```python
from build123d import *

# Parameters (mm, degrees)
SKETCH1_R               = 2.85
SKETCH1_R_2             = 1.6
BOSS_EXTRUDE1_DEPTH     = 6.5
SKETCH1_3_R             = 2.85
SKETCH1_3_R_2           = 1.6
BOSS_EXTRUDE2_DEPTH     = 3
CUT_EXTRUDE1_START      = -3
SKETCH1_4_R             = 2.85
CUT_EXTRUDE1_DEPTH      = 3.5
CUT_EXTRUDE1_DEPTH_BACK = 4


with BuildPart() as part:
    # Sketch1 → Boss-Extrude1 (new body)
    with BuildSketch(Plane(origin=(0, 0, 0), x_dir=(0, 1, 0), z_dir=(0, 0, 1))):
        Polygon((-7.9, 10.1), (-9.9, 10.1), (-9.9, 0), (-9.1, 0), (-9.1, -2), (-20.1, -2), (-20.1, 11.6), (-7.9, 11.6), align=None)
        with Locations((-14.9, 6.1)):
            Circle(SKETCH1_R, mode=Mode.SUBTRACT)
        Polygon((13.4, 11.6), (20.1, 11.6), (20.1, -2), (9.1, -2), (9.1, 0), (9.9, 0), (9.9, 9.3), (6.4, 9.3), (6.4, 10.8), (13.4, 10.8), align=None)
        with Locations((14.9, 6.1)):
            Circle(SKETCH1_R, mode=Mode.SUBTRACT)
        with Locations((-14.9, 6.1)):
            Circle(SKETCH1_R)
        with Locations((-14.9, 6.1)):
            Circle(SKETCH1_R_2, mode=Mode.SUBTRACT)
        with Locations((14.9, 6.1)):
            Circle(SKETCH1_R)
        with Locations((14.9, 6.1)):
            Circle(SKETCH1_R_2, mode=Mode.SUBTRACT)
    extrude(amount=BOSS_EXTRUDE1_DEPTH)

    # Sketch1<3> → Boss-Extrude2 (add)
    with BuildSketch(Plane(origin=(0, 0, 0), x_dir=(0, 1, 0), z_dir=(0, 0, 1))):
        with Locations((14.9, 6.1)):
            Circle(SKETCH1_3_R)
        with Locations((14.9, 6.1)):
            Circle(SKETCH1_3_R_2, mode=Mode.SUBTRACT)
        Polygon((13.4, 11.6), (20.1, 11.6), (20.1, -2), (9.1, -2), (9.1, 0), (9.9, 0), (9.9, 9.3), (6.4, 9.3), (6.4, 10.8), (13.4, 10.8), align=None)
        with Locations((14.9, 6.1)):
            Circle(SKETCH1_3_R, mode=Mode.SUBTRACT)
        Polygon((-7.9, 11.6), (13.4, 11.6), (13.4, 10.8), (6.4, 10.8), (6.4, 9.3), (9.9, 9.3), (9.9, 0), (9.1, 0), (9.1, -2), (-9.1, -2), (-9.1, 0), (-9.9, 0), (-9.9, 10.1), (-7.9, 10.1), align=None)
        with Locations((-14.9, 6.1)):
            Circle(SKETCH1_3_R)
        with Locations((-14.9, 6.1)):
            Circle(SKETCH1_3_R_2, mode=Mode.SUBTRACT)
        Polygon((-7.9, 10.1), (-9.9, 10.1), (-9.9, 0), (-9.1, 0), (-9.1, -2), (-20.1, -2), (-20.1, 11.6), (-7.9, 11.6), align=None)
        with Locations((-14.9, 6.1)):
            Circle(SKETCH1_3_R, mode=Mode.SUBTRACT)
    extrude(amount=-BOSS_EXTRUDE2_DEPTH)

    # Sketch1<4> → Cut-Extrude1 (cut, two sides)
    with BuildSketch(Plane(origin=(0, 0, 0), x_dir=(0, 1, 0), z_dir=(0, 0, 1)).offset(CUT_EXTRUDE1_START)) as cut_extrude1_sk:
        with Locations((14.9, 6.1)):
            Circle(SKETCH1_4_R)
        with Locations((-14.9, 6.1)):
            Circle(SKETCH1_4_R)
    extrude(amount=CUT_EXTRUDE1_DEPTH, mode=Mode.SUBTRACT)
    extrude(cut_extrude1_sk.sketch, amount=-CUT_EXTRUDE1_DEPTH_BACK, mode=Mode.SUBTRACT)


solid = part.part
```
Model file for the job. Use its own axes, mm. A direction names the side the tool comes from. Coordinates: 2 decimals unless noted, no trailing zeros. Write each loop counter-clockwise with the first axis right and the second up, starting at its lowest first coordinate (ties: lowest second). Pieces come first, ordered by that corner, then holes. Notation, with made-up numbers: (52.5, -3) - (58.5, -3) arc R18 cw to (58.5, 4) - close; hole circle Ø10 at (-13, 68). An arc over 180 degrees is marked (long way). One line per item, written item: value. Start each with the question number.
1. Slice it at D-D (x = -0.75). Write the cut outline in (y, z), plus the area to 3 significant figures.
2. Mould opens along X. For faces 1 (the flat face through (-9.3, 8, 3)), 2 (the flat face through (-5, 0, -3)), 3 (the flat face through (-10.8, 10, 3)) say: released by +X, released by -X, zero draft, split by the parting line, or undercut.
3. Slice it at B-B (z = 5). Write the cut outline in (x, y), plus the area to 3 significant figures.
4. Slice it at A-A (x = -6.1). Write the cut outline in (y, z).
5. Slice it at C-C (y = -14.9). Write the cut outline in (x, z).
6. Tool access for faces 4 (the flat face through (-5, -20.1, 2)), 5 (the flat face through (1, -9.1, 3)), 6 (the flat face through (-10, 6.4, 3)), 7 (the flat face through (0, -9.5, 3.2)), 8 (the cylindrical face through (-6.956, 17.618, -1.226)): list every direction of +Z, -Z, +X, -X, +Y, -Y with a clear straight run to the whole face (end or side of a thin tool).
7. Flat gauge pins, fed straight in: pin 1 (7.5 mm diameter, centred on x = -6.1, y = -14.9, fed in from -Z); pin 2 (2.5 mm diameter, centred on x = -6.1, y = -14.9, fed in from -Z). Where does each tip first touch, or does it go through?
8. Probe line 1 (Y direction, x = -6.1, z = -0.6); line 2 (Y direction, x = -6.1, z = 5.15); line 3 (Y direction, x = -2.5, z = 2.5). List the from-to ranges inside material, lowest first. Write a range as from..to.
Answers below:
1. outline: (-20.1, -3) - (20.1, -3) - (20.1, 6.5) - (9.9, 6.5) - (9.9, 0) - (-9.9, 0) - (-9.9, 6.5) - (-20.1, 6.5) - close
1. area: 253 mm^2
2. face 1: undercut
2. face 2: zero draft
2. face 3: released by -X
3. outline: (-11.6, -20.1) - (2, -20.1) - (2, -9.1) - (0, -9.1) - (0, -9.9) - (-10.1, -9.9) - (-10.1, -7.9) - (-11.6, -7.9) - close; (-11.6, 13.4) - (-10.8, 13.4) - (-10.8, 6.4) - (-9.3, 6.4) - (-9.3, 9.9) - (0, 9.9) - (0, 9.1) - (2, 9.1) - (2, 20.1) - (-11.6, 20.1) - close; hole circle Ø3.2 at (-6.1, -14.9); hole circle Ø3.2 at (-6.1, 14.9)
3. area: 270 mm^2
4. outline: (-20.1, -3) - (-17.75, -3) - (-17.75, 0.5) - (-16.5, 0.5) - (-16.5, 6.5) - (-20.1, 6.5) - close; (-13.3, 0.5) - (-12.05, 0.5) - (-12.05, -3) - (12.05, -3) - (12.05, 0.5) - (13.3, 0.5) - (13.3, 6.5) - (9.9, 6.5) - (9.9, 0) - (-9.9, 0) - (-9.9, 6.5) - (-13.3, 6.5) - close; (16.5, 0.5) - (17.75, 0.5) - (17.75, -3) - (20.1, -3) - (20.1, 6.5) - (16.5, 6.5) - close
5. outline: (-11.6, -3) - (-8.95, -3) - (-8.95, 0.5) - (-7.7, 0.5) - (-7.7, 6.5) - (-11.6, 6.5) - close; (-4.5, 0.5) - (-3.25, 0.5) - (-3.25, -3) - (2, -3) - (2, 6.5) - (-4.5, 6.5) - close
6. face 4: +Z, -Z, +X, -X, -Y
6. face 5: +Z, +X
6. face 6: +Z, +X, -X
6. face 7: +Z
6. face 8: -Z
7. pin 1: stops at z = -3
7. pin 2: passes through
8. line 1: y = -20.1..-17.75, -12.05..12.05, 17.75..20.1
8. line 2: y = -20.1..-16.5, -13.3..-9.9, 9.9..13.3, 16.5..20.1
8. line 3: y = -20.1..-9.9, 9.9..20.1
